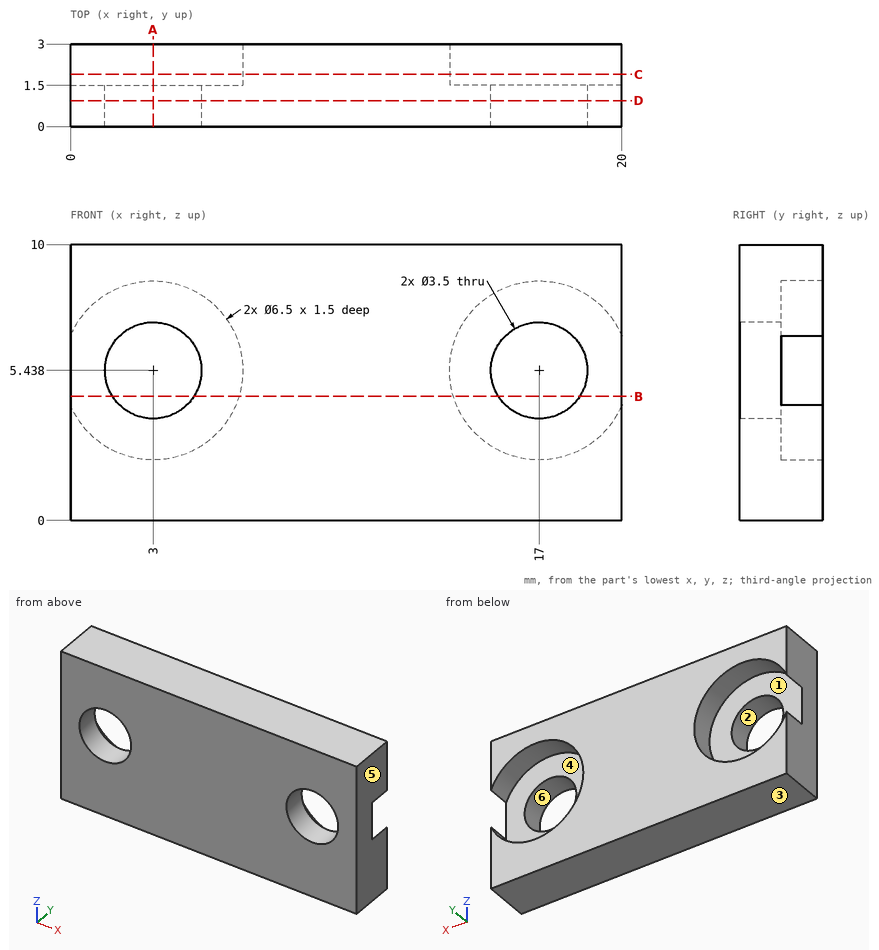
Design review of the part shown in the three views and the two pictorial views. Dimensions are in mm from the part's minimum x, y and z. A direction names the side the tool comes from. Coordinates: 2 decimals unless noted, no trailing zeros. Write each loop counter-clockwise with the first axis right and the second up, starting at its lowest first coordinate (ties: lowest second). Pieces come first, ordered by that corner, then holes.
1) The part is to be moulded in two halves that separate along Z. For the marked faces 3, 4, 5 and 6, say which applies: pulls with the +Z half, pulls with the -Z half, needs draft (parallel to the pull), parting line crosses it, or undercut.
2) To check wall thickness, follow probe 1 along X at (y, z) = (2.3, 7.75) (1 decimal); probe 2 along Z at (x, y) = (3, 2.6); probe 3 along X at (y, z) = (0.8, 5.75). State the ranges of each line that lie inside material, in increasing order.
3) We need section D-D on y = 0.95. State the section outline as (x, z) points, then the cut area to 3 significant figures.
4) We need section C-C on y = 1.9. State the section outline as (x, z) points.
5) Machinability: for the marked faces 1 and 2, which of the approach directions +Z, -Z, +X, -X, +Y, -Y give a long, thin tool a straight path to every point of the face, cutting with its end or side? Answer none if there is none.
6) We need section A-A on x = 3. State the section outline as (y, z) points, then the cut area to 3 significant figures.
7) We need section B-B on z = 4.5. State the section outline as (x, y) points, then the cut area to 3 significant figures.
8) Clearance check with a flat-ended pin moving along its axis: pin 1 Ø3 at (x, z) = (15.5, 5.5) entering from +Y. State where the tip first meets the part, or that it passes through.
Answer list:
1. face 3: pulls with the -Z half
1. face 4: undercut
1. face 5: needs draft
1. face 6: undercut
2. probe 1: x = 0 to 0.7, 5.3 to 14.7, 19.3 to 20
2. probe 2: z = 0 to 2.19, 8.69 to 10
2. probe 3: x = 0 to 1.28, 4.72 to 15.28, 18.72 to 20
3. outline: (0, 0) - (20, 0) - (20, 10) - (0, 10) - close; hole circle Ø3.5 at (3, 5.44); hole circle Ø3.5 at (17, 5.44)
3. area: 181 mm2
4. outline: (0, 0) - (20, 0) - (20, 4.19) arc R3.25 cw (long way) to (20, 6.69) - (20, 10) - (0, 10) - (0, 6.69) arc R3.25 cw (long way) to (0, 4.19) - close
5. face 1: +Y
5. face 2: +Y, -Y
6. outline: (0, 0) - (3, 0) - (3, 2.19) - (1.5, 2.19) - (1.5, 3.69) - (0, 3.69) - close; (0, 7.19) - (1.5, 7.19) - (1.5, 8.69) - (3, 8.69) - (3, 10) - (0, 10) - close
6. area: 15.0 mm2
7. outline: (0, 0) - (1.52, 0) - (1.52, 1.5) - (0, 1.5) - close; (4.48, 0) - (15.52, 0) - (15.52, 1.5) - (13.89, 1.5) - (13.89, 3) - (6.11, 3) - (6.11, 1.5) - (4.48, 1.5) - close; (18.48, 0) - (20, 0) - (20, 1.5) - (18.48, 1.5) - close
7. area: 32.8 mm2
8. pin 1: stops at y = 1.5
